Verification items for the finished model (mm, model axes). A direction names the side the tool comes from. Round coordinates to 2 decimals unless told otherwise and drop trailing zeros. Write each loop counter-clockwise with the first axis right and the second up, starting at its lowest first coordinate (ties: lowest second). Pieces come first, ordered by that corner, then holes. Notation, with made-up numbers: M 57.25,-17.5 L 68.25,-17.5 A36 cw 68.25,16.5 Z; hole C -38.75,-11 d7. An arc over 180 degrees is marked long. Answer in a Markdown table with one row per item. Add a question column.
1. Sectioned sample at A-A on y = -33. Record the cut outline in (x, z) (3 decimals), plus the area to 3 significant figures.
2. Set-up check for faces 5 (the flat face through (0, -38.1, 4)), 6 (the flat face through (-32, -10, 2.794)), 7 (the flat face through (0, 31.75, 6)): record each of +Z, -Z, +X, -X, +Y, -Y from which the full face is reachable in a straight line by a thin tool's end or side.
3. Draft check along X on faces 1 (the flat face through (0, -31.75, -7)), 2 (the flat face through (-34, 1, 9.525)), 3 (the flat face through (38.1, 0, 0)), 4 (the flat face through (-38.1, 0, 0)). Enter one of: pulls with the +X half, pulls with the -X half, needs draft (parallel to the pull), parting line crosses it, or undercut.
4. Go/stop test with a flat-tipped pin: pin 1 Ø0.5 at (x, z) = (10, 2.5) entering from -Y. Record where the tip stops, or that it passes through.
5. Material ranges on probe 1 along X at (y, z) = (-9, -1); probe 2 along X at (y, z) = (24, 0), recorded low to high.
6. Sectioned sample at B-B on z = 7.75. Record the cut outline in (x, y) (3 decimals).
7. Sectioned sample at C-C on x = 1. Count the separate pieces of the cut face and the enclosed holes in it, plus the area to 3 significant figures.
```python
from build123d import *

# Parameters (mm, degrees)
F0_W     = 76.2
F0_H     = 76.2
F0_W_2   = 63.5
F0_H_2   = 63.5
F1_DEPTH = 9.525
F2_W     = 66.04
F2_H     = 1.016
F3_DEPTH = 38.1
F4_DEPTH = 31.75
F5_R     = 3.175
F6_DEPTH = 33.02


with BuildPart() as f1:
    # F0 (on Top) → F1 (new body, symmetric)
    with BuildSketch(Plane.XY):
        Rectangle(F0_W, F0_H)
        Rectangle(F0_W_2, F0_H_2, mode=Mode.SUBTRACT)
    extrude(amount=F1_DEPTH, both=True)

    # F2 (on Front) → F3 (cut, through all)
    with BuildSketch(Plane.XZ):
        Rectangle(F2_W, F2_H)
        with Locations((0, 2.286)):
            Rectangle(F2_W, F2_H)
        with Locations((0, -2.286)):
            Rectangle(F2_W, F2_H)
        with Locations((0, -4.572)):
            Rectangle(F2_W, F2_H)
    extrude(amount=F3_DEPTH, mode=Mode.SUBTRACT)

    # F2 (on Front) → F4 (cut)
    with BuildSketch(Plane.XZ):
        Rectangle(F2_W, F2_H)
        with Locations((0, 2.286)):
            Rectangle(F2_W, F2_H)
        with Locations((0, -2.286)):
            Rectangle(F2_W, F2_H)
        with Locations((0, -4.572)):
            Rectangle(F2_W, F2_H)
    extrude(amount=-F4_DEPTH, mode=Mode.SUBTRACT)

    # F5
    f5_edges = [f1.edges().sort_by_distance(p)[0] for p in [
        (-38.1, -38.1, 0),
        (38.1, -38.1, 0),
        (38.1, 38.1, 0),
        (-38.1, 38.1, 0),
    ]]
    fillet(f5_edges, radius=F5_R)

    # F2 (on Front) → F6 (cut)
    with BuildSketch(Plane.XZ):
        Rectangle(F2_W, F2_H)
        with Locations((0, 2.286)):
            Rectangle(F2_W, F2_H)
        with Locations((0, -2.286)):
            Rectangle(F2_W, F2_H)
        with Locations((0, -4.572)):
            Rectangle(F2_W, F2_H)
    extrude(amount=-F6_DEPTH, mode=Mode.SUBTRACT)


solid = f1.part
```
Geometry check:
| question | item | result |
|---|---|---|
| 1 | outline | M -38.1,-9.525 L 38.1,-9.525 L 38.1,9.525 L -38.1,9.525 Z; hole M -33.02,-5.08 L 33.02,-5.08 L 33.02,-4.064 L -33.02,-4.064 Z; hole M -33.02,-2.794 L 33.02,-2.794 L 33.02,-1.778 L -33.02,-1.778 Z; hole M -33.02,-0.508 L 33.02,-0.508 L 33.02,0.508 L -33.02,0.508 Z; hole M -33.02,1.778 L 33.02,1.778 L 33.02,2.794 L -33.02,2.794 Z |
| 1 | area | 1,180 mm2 |
| 2 | face 5 | +Z, -Z, +X, -X, -Y |
| 2 | face 6 | -Y |
| 2 | face 7 | +Z, -Z |
| 3 | face 1 | undercut |
| 3 | face 2 | needs draft |
| 3 | face 3 | pulls with the +X half |
| 3 | face 4 | pulls with the -X half |
| 4 | pin 1 | stops at y = 33.02 |
| 5 | probe 1 | x = -38.1 to -31.75, 31.75 to 38.1 |
| 5 | probe 2 | x = -38.1 to -33.02, 33.02 to 38.1 |
| 6 | outline | M -38.1,-34.925 A3.175 ccw -34.925,-38.1 L 34.925,-38.1 A3.175 ccw 38.1,-34.925 L 38.1,34.925 A3.175 ccw 34.925,38.1 L -34.925,38.1 A3.175 ccw -38.1,34.925 Z; hole M -31.75,-31.75 L 31.75,-31.75 L 31.75,31.75 L -31.75,31.75 Z |
| 7 | separate pieces | 6 |
| 7 | enclosed holes | 0 |
| 7 | area | 211 mm2 |
